Work out the finished part from the listing and answer in its coordinate system (mm). Face numbers are marked on the shaded views. A direction names the side the tool comes from. Give positions to 0.01 mm unless a question says otherwise; leave off trailing zeros. Loops run counter-clockwise (first coordinate to the right, second up) from the corner with the lowest first, then second, coordinate; pieces in that order, holes last. Notation, with made-up numbers: (1.25, 71) - (53.25, 71) arc R9 cw to (53.25, 83) - close; hole circle Ø2 at (4, 79.5). An arc over 180 degrees is marked (long way). One line per item, written item: value.
from build123d import *

# Parameters (mm, degrees)
SALIENTE_EXTRUIR1_DEPTH = 10
CROQUIS2_R              = 1.5
CORTAR_EXTRUIR1_DEPTH   = 10
CROQUIS3_W              = 15
CROQUIS3_H              = 2.5
CORTAR_EXTRUIR2_DEPTH   = 10
CROQUIS4_R              = 1.5
CORTAR_EXTRUIR3_DEPTH   = 10
CORTAR_EXTRUIR5_DEPTH   = 10
CROQUIS9_R              = 2
SALIENTE_EXTRUIR2_DEPTH = 2.5
CROQUIS10_W             = 80
CROQUIS10_H             = 16.68210675
CROQUIS10_H_2           = 15.952607418
CORTAR_EXTRUIR6_DEPTH   = 10
REDONDEO1_R             = 5


with BuildPart() as part:
    # Croquis1 → Saliente-Extruir1 (new body)
    with BuildSketch(Plane.XY):
        Polygon((0, 0), (105, 0), (105, 2.5), (105, 7.5), (105, 10), (0, 10), (0, 7.5), (15, 7.5), (15, 2.5), (0, 2.5), align=None)
    extrude(amount=SALIENTE_EXTRUIR1_DEPTH)

    # Croquis2 → Cortar-Extruir1 (cut)
    with BuildSketch(Plane(origin=(0, 10, 0), x_dir=(1, 0, 0), z_dir=(0, 1, 0))):
        with Locations(Location((5, -5, 0), (0, 0, 270))):
            Circle(CROQUIS2_R)
        with BuildLine():
            Line((-4.031911586, 0), (5, 0))
            ThreePointArc((5, 0), (0, -5), (5, -10))
            Line((5, -10), (-4.031911586, -10))
            Line((-4.031911586, -10), (-4.031911586, 0))
        make_face()
    extrude(amount=-CORTAR_EXTRUIR1_DEPTH, mode=Mode.SUBTRACT)

    # Croquis3 → Cortar-Extruir2 (cut)
    with BuildSketch(Plane(origin=(0, 10, 0), x_dir=(1, 0, 0), z_dir=(0, 1, 0))):
        with Locations((97.5, -1.25)):
            Rectangle(CROQUIS3_W, CROQUIS3_H)
        with Locations((97.5, -8.75)):
            Rectangle(CROQUIS3_W, CROQUIS3_H)
    extrude(amount=-CORTAR_EXTRUIR2_DEPTH, mode=Mode.SUBTRACT)

    # Croquis4 → Cortar-Extruir3 (cut)
    with BuildSketch(Plane.XY.offset(7.5)):
        with Locations((100, 5)):
            Circle(CROQUIS4_R)
        with BuildLine():
            Line((100, 10), (171.112400038, 10))
            Line((171.112400038, 10), (171.112400038, 0))
            Line((171.112400038, 0), (100, 0))
            ThreePointArc((100, 0), (105, 5), (100, 10))
        make_face()
    extrude(amount=-CORTAR_EXTRUIR3_DEPTH, mode=Mode.SUBTRACT)

    # Croquis8 → Cortar-Extruir5 (cut)
    with BuildSketch(Plane.XY.offset(7.5)):
        with BuildLine():
            Line((90, 0), (100, 0))
            ThreePointArc((100, 0), (105, 5), (100, 10))
            Line((100, 10), (90, 10))
            Line((90, 10), (90, 0))
        make_face()
    extrude(amount=-CORTAR_EXTRUIR5_DEPTH, mode=Mode.SUBTRACT)

    # Croquis9 → Saliente-Extruir2 (add, symmetric)
    with BuildSketch(Plane(origin=(0, 5, 0), x_dir=(-1, 0, 0), z_dir=(0, -1, 0))):
        with BuildLine():
            Line((-90, -10), (-95, -10))
            ThreePointArc((-95, -10), (-100, -5), (-95, 0))
            Line((-95, 0), (-90, 0))
            Line((-90, 0), (-90, -10))
        make_face()
        with Locations(Location((-95, -5, 0), (0, 0, 90))):
            Circle(CROQUIS9_R, mode=Mode.SUBTRACT)
    extrude(amount=SALIENTE_EXTRUIR2_DEPTH, both=True)

    # Croquis10 → Cortar-Extruir6 (cut)
    with BuildSketch(Plane(origin=(0, 0, 0), x_dir=(-1, 0, 0), z_dir=(0, 0, -1))):
        with Locations((-60, 15.841053375)):
            Rectangle(CROQUIS10_W, CROQUIS10_H)
        with Locations((-60, -5.476303709)):
            Rectangle(CROQUIS10_W, CROQUIS10_H_2)
    extrude(amount=-CORTAR_EXTRUIR6_DEPTH, mode=Mode.SUBTRACT)

    # Redondeo1
    # the kernel refuses this fillet: 5 mm, written as the material it adds along each edge
    with BuildSketch(Plane(origin=(20, 2.5, 0), x_dir=(1, 0, 0), z_dir=(0, 0, 1))) as redondeo1_piece_1:
        with BuildLine():
            CenterArc((4.330127019, -5), REDONDEO1_R, 90, 60)
            Line((0, -2.5), (-0.08660254, -2.45))
            ThreePointArc((-0.08660254, -2.45), (-0.1, -1.25), (-0.1, 0))
            Line((-0.1, 0), (0, 0.1))
            Line((0, 0.1), (4.330127019, 0.1))
            Line((4.330127019, 0.1), (4.330127019, 0))
        make_face()
    extrude(amount=10)
    with BuildSketch(Plane(origin=(20, 7.5, 0), x_dir=(0, 1, 0), z_dir=(0, 0, 1))) as redondeo1_piece_2:
        with BuildLine():
            CenterArc((5, -4.330127019), REDONDEO1_R, 120, 60)
            Line((0, -4.330127019), (-0.1, -4.330127019))
            Line((-0.1, -4.330127019), (-0.1, 0))
            Line((-0.1, 0), (0, 0.1))
            ThreePointArc((0, 0.1), (1.25, 0.1), (2.45, 0.08660254))
            Line((2.45, 0.08660254), (2.5, 0))
        make_face()
    extrude(amount=10)


solid = part.part
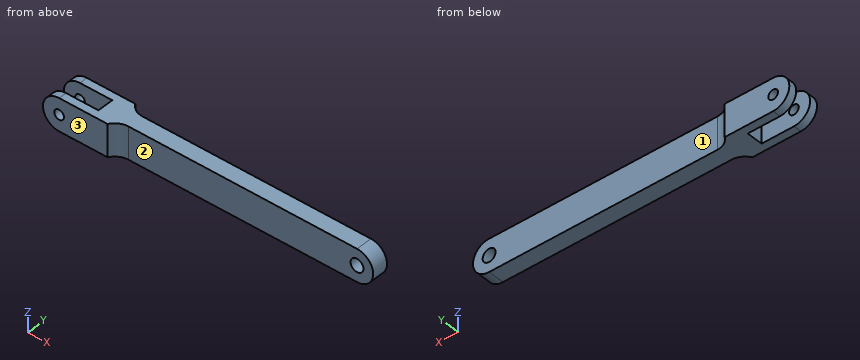
1. For the marked faces 1, 2 and 3, determine the directions among +Z, -Z, +X, -X, +Y, -Y from which every point of the face is accessible in a straight line to the end or side of a thin tool.
Output:
face 1: +Z, -Z, +X, +Y
face 2: +Z, -Z, +X, -Y
face 3: +Z, -Z, +X, -X, -Y
2. Section B-B (x = 9.5) is taken. Write down the section's boundary in (y, z).
Output:
outline: (0, 0) - (2.5, 0) - (2.5, 10) - (0, 10) - close; (7.5, 0) - (10, 0) - (10, 10) - (7.5, 10) - close
3. Section A-A (z = 5) is taken. Write down the section's boundary in (x, y), and give its area (3 significant figures).
Output:
outline: (0, 0) - (3.5, 0) - (3.5, 2.5) - (0, 2.5) - close; (0, 7.5) - (3.5, 7.5) - (3.5, 10) - (0, 10) - close; (6.5, 0) - (20, 0) arc R5 cw to (24.33, 2.5) - (93, 2.5) - (93, 7.5) - (24.33, 7.5) arc R5 cw to (20, 10) - (6.5, 10) - (6.5, 7.5) - (15, 7.5) - (15, 2.5) - (6.5, 2.5) - close; (97, 2.5) - (100, 2.5) - (100, 7.5) - (97, 7.5) - close
area: 496 mm²
4. Section C-C (y = 5.5) is taken. Write down the section's boundary in (x, z), and give its area (3 significant figures).
Output:
outline: (15, 0) - (95, 0) arc R5 ccw to (95, 10) - (15, 10) - close; hole circle Ø4 at (95, 5)
area: 827 mm²
5. Flat-ended cylindrical pins translate along their axes: pin 1 Ø3 at (y, z) = (7, 2) entering from -X; pin 2 Ø1.5 at (y, z) = (6.5, 8) entering from +X; pin 3 Ø2.5 at (y, z) = (5, 2.5) entering from -X. Find the tip coordinate at first contact, or state that the pin passes through.
Output:
pin 1: stops at x = 0.26
pin 2: stops at x = 99.47
pin 3: stops at x = 15
6. Find the intervals of material crossed by line 1 along Y through (x, z) = (6, 1); line 2 along Y through (x, z) = (76, 3.5); line 3 along X through (y, z) = (9.25, 5), in increasing order.
Output:
line 1: y = 0 to 2.5, 7.5 to 10
line 2: y = 2.5 to 7.5
line 3: x = 0 to 3.5, 6.5 to 20.53
7. Section D-D (x = 62) is taken. Write down the section's boundary in (y, z), and give its area (3 significant figures).
Output:
outline: (2.5, 0) - (7.5, 0) - (7.5, 10) - (2.5, 10) - close
area: 50.0 mm²
